from build123d import *

# Parameters (mm, degrees)
SKETCH1_R                  = 90
SKETCH1_R_2                = 30
BOSS_EXTRUDE1_DEPTH        = 8
SKETCH2_R                  = 50
SKETCH2_R_2                = 30
BOSS_EXTRUDE2_DEPTH        = 10
F_12_0_12_DIAMETER_HOLE1_D = 12


with BuildPart() as part:
    # Sketch1 → Boss-Extrude1 (new, symmetric)
    with BuildSketch(Plane.XY):
        Circle(SKETCH1_R)
        with Locations((-2.481799725, 0)):
            Circle(SKETCH1_R_2, mode=Mode.SUBTRACT)
    extrude(amount=BOSS_EXTRUDE1_DEPTH, both=True)

    # Sketch2 → Boss-Extrude2 (add)
    with BuildSketch(Plane.XY.offset(8)):
        Circle(SKETCH2_R)
        with Locations((-2.481799725, 0)):
            Circle(SKETCH2_R_2, mode=Mode.SUBTRACT)
    extrude(amount=BOSS_EXTRUDE2_DEPTH)

    # Ø12.0 (12) Diameter Hole1 (through all)
    with Locations(Plane(origin=(0, 40, 18), x_dir=(1, 0, 0), z_dir=(0, 0, 1))):
        with Locations((0, 0), (-38.042260652, -27.639320225), (-23.511410092, -72.360679775), (23.511410092, -72.360679775), (38.042260652, -27.639320225)):
            Hole(F_12_0_12_DIAMETER_HOLE1_D / 2)


solid = part.part
CAD build for the part. Positions are in the model's coordinates, mm. A direction names the side the tool comes from. Round coordinates to 2 decimals unless told otherwise and drop trailing zeros. Loops run counter-clockwise (first coordinate to the right, second up) from the corner with the lowest first, then second, coordinate; pieces in that order, holes last. Notation, with made-up numbers: M 78,14.5 L 124,14.5 A18 cw 124,45.5 Z; hole C 51.25,-28 d8. An arc over 180 degrees is marked long. One line per question, with ' | ' between items. Start each with the question number.
Item 1: Pin check, flat tips, straight feed: pin 1 Ø2 at (x, z) = (-27.5, 11.5) entering from +Y; pin 2 Ø12 at (x, y) = (36, -63) entering from +Z; pin 3 Ø6 at (x, z) = (-23.5, 12) entering from +Y; pin 4 Ø7 at (x, y) = (-38.04, 12.36) entering from -Z. Stop position of each tip, or through.
Item 2: Cut at A-A, the plane y = 0. Write the cut outline in (x, z), plus the area to 3 significant figures.
Item 3: Which spindle directions (+Z, -Z, +X, -X, +Y, -Y) get a long thin tool onto all of the face, cutting with end or side? Do faces 1 (the flat face through (39, -39, 8)), 2 (the cylindrical face through (-22.73, -26.41, 4.82)). Say none if no direction does.
Item 4: Wall check: line 1 (Y direction, x = -20.5, z = 10.75); line 2 (Z direction, x = -52, y = 22); line 3 (X direction, y = 12, z = 9.5). Give the ranges that are in metal, low to high.
Item 5: Two-plate mould, pull along X, no slides. Class faces 3 (the flat face through (22, -22, 18)), 4 (the cylindrical face through (-43.6, 10.1, 4.8)), 5 (the cylindrical face through (41.53, -79.845, 0.112)): pulls with the +X half, pulls with the -X half, needs draft (parallel to the pull), parting line crosses it, or undercut.
Item 6: Cut at B-B, the plane x = 0. Write the cut outline in (y, z), plus the area to 3 significant figures.
Item 7: Cut at D-D, the plane y = -78.5. Write the cut outline in (x, z).
Item 8: Cut at C-C, the plane z = 12.5. Write the cut outline in (x, y), plus the area to 3 significant figures.
Responses:
1) pin 1: stops at y = 42.4 | pin 2: stops at z = 8 | pin 3: stops at y = 45.6 | pin 4: passes through
2) outline: M -90,-8 L -32.48,-8 L -32.48,18 L -50,18 L -50,8 L -90,8 Z; M 27.52,-8 L 90,-8 L 90,8 L 50,8 L 50,18 L 27.52,18 Z | area: 2,320 mm²
3) face 1: +Z | face 2: +Z, -Z
4) line 1: y = -45.6 to -37.55, -27.17 to -23.99, 23.99 to 45.6 | line 2: z = -8 to 8 | line 3: x = -48.54 to -44.03, -32.05 to -29.98, 25.01 to 32.05, 44.03 to 48.54
5) face 3: needs draft | face 4: undercut | face 5: parting line crosses it
6) outline: M -90,-8 L -29.9,-8 L -29.9,18 L -50,18 L -50,8 L -90,8 Z; M 29.9,-8 L 34,-8 L 34,18 L 29.9,18 Z; M 46,-8 L 90,-8 L 90,8 L 50,8 L 50,18 L 46,18 Z | area: 2,010 mm²
7) outline: M -44.02,-8 L 44.02,-8 L 44.02,8 L -44.02,8 Z
8) outline: C 0,0 d100; hole C -38.04,12.36 d12; hole C -2.48,0 d60; hole C -23.51,-32.36 d12; hole C 0,40 d12; hole C 23.51,-32.36 d12; hole C 38.04,12.36 d12 | area: 4,460 mm²
